Geometry: final body of the model. Coordinates: model frame, mm. Coordinates: 2 decimals unless noted, no trailing zeros. Use one line per item in the form item = value. Start each with the question number.
```python
from build123d import *

# Parameters (mm, degrees)
F0_W     = 15
F0_H     = 10
F0_W_2   = 30
F1_DEPTH = 10
F3_D     = 1.5
F3_DEPTH = 5
F2_R     = 0.75
F4_DEPTH = 25


with BuildPart() as f1:
    # F0 (on Front) → F1 (new body)
    with BuildSketch(Plane.XZ):
        with Locations((-53.005068, 3.119589)):
            Rectangle(F0_W, F0_H)
        with Locations((-30.505068, 3.119589)):
            Rectangle(F0_W_2, F0_H)
        with Locations((-8.005068, 3.119589)):
            Rectangle(F0_W, F0_H)
    extrude(amount=F1_DEPTH)

    # F3
    with Locations(Plane.XZ.offset(10)):
        with Locations((-45.505068, 3.119589)):
            Hole(F3_D / 2, depth=F3_DEPTH)

    # F2 (on face) → F4 (cut)
    with BuildSketch(Plane.XZ.offset(10)):
        with Locations((-45.505068, 3.119589)):
            Circle(F2_R)
        with Locations((-15.505068, 3.119589)):
            Circle(F2_R)
    extrude(amount=-F4_DEPTH, mode=Mode.SUBTRACT)


solid = f1.part
```
(1) Draft query along X for faces 1 (the flat face through (-31, -5, -1.88)), 2 (the flat face through (-0.505, -5, 3)), 3 (the cylindrical face through (-14.812, -5.07, 2.832)). Return one class per face: released by +X, released by -X, zero draft, split by the parting line, or undercut.
(2) Contact query for a flat-ended pin moving along its axis: pin 1 Ø0.9 at (x, z) = (-45.51, 3.12) entering from +Y. Output: stop coordinate, or through.
(3) Material intervals for L1, parallel to X at y = -2, z = 3.5; L2, parallel to X at y = -5.5, z = 2.5, sorted ascending. Write a range as from..to.
Check sheet entries:
q1.face_1 = zero draft
q1.face_2 = released by +X
q1.face_3 = undercut
q2.pin_1 = through
q3.L1 = -60.51..-46.15, -44.86..-16.15, -14.86..-0.51
q3.L2 = -60.51..-45.93, -45.08..-15.93, -15.08..-0.51
